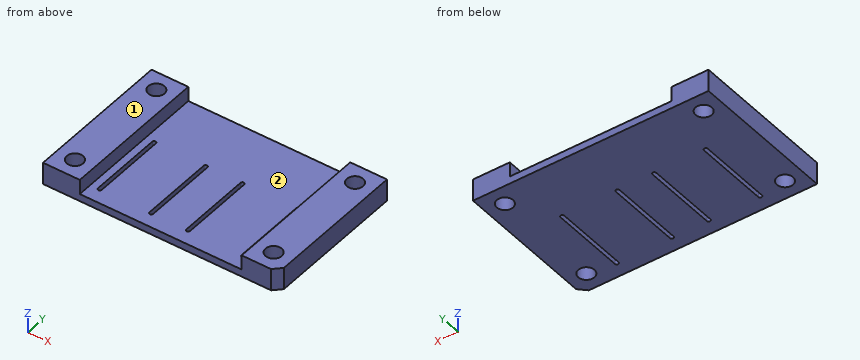
from build123d import *

# Parameters (mm, degrees)
SKETCH1_W           = 320
SKETCH1_H           = 200
SKETCH1_R           = 11
BOSS_EXTRUDE1_DEPTH = 30
CUT_EXTRUDE1_DEPTH  = 379.549864615
SKETCH4_W           = 220
SKETCH4_H           = 200
CUT_EXTRUDE2_DEPTH  = 20
CHAMFER1_SIZE       = 10


with BuildPart() as part:
    # Sketch1 → Boss-Extrude1 (new body)
    with BuildSketch(Plane.XY):
        with Locations((160, 100)):
            Rectangle(SKETCH1_W, SKETCH1_H)
        with Locations((25, 175)):
            Circle(SKETCH1_R, mode=Mode.SUBTRACT)
        with Locations((295, 175)):
            Circle(SKETCH1_R, mode=Mode.SUBTRACT)
        with Locations((25, 25)):
            Circle(SKETCH1_R, mode=Mode.SUBTRACT)
        with Locations((295, 25)):
            Circle(SKETCH1_R, mode=Mode.SUBTRACT)
    extrude(amount=BOSS_EXTRUDE1_DEPTH)

    # Sketch2 → Cut-Extrude1 (cut, through all)
    with BuildSketch(Plane.XY.offset(30)):
        with BuildLine():
            Line((260, 120), (260, 20))
            ThreePointArc((260, 20), (257.5, 17.5), (255, 20))
            Line((255, 20), (255, 120))
            ThreePointArc((255, 120), (257.5, 122.5), (260, 120))
        make_face()
        with BuildLine():
            Line((185, 120), (185, 20))
            ThreePointArc((185, 20), (182.5, 17.5), (180, 20))
            Line((180, 20), (180, 120))
            ThreePointArc((180, 120), (182.5, 122.5), (185, 120))
        make_face()
        with BuildLine():
            Line((65, 120), (65, 20))
            ThreePointArc((65, 20), (62.5, 17.5), (60, 20))
            Line((60, 20), (60, 120))
            ThreePointArc((60, 120), (62.5, 122.5), (65, 120))
        make_face()
        with BuildLine():
            Line((135, 120), (135, 20))
            ThreePointArc((135, 20), (132.5, 17.5), (130, 20))
            Line((130, 20), (130, 120))
            ThreePointArc((130, 120), (132.5, 122.5), (135, 120))
        make_face()
    extrude(amount=-CUT_EXTRUDE1_DEPTH, mode=Mode.SUBTRACT)

    # Sketch4 → Cut-Extrude2 (cut)
    with BuildSketch(Plane.XY.offset(30)):
        with Locations((160, 100)):
            Rectangle(SKETCH4_W, SKETCH4_H)
    extrude(amount=-CUT_EXTRUDE2_DEPTH, mode=Mode.SUBTRACT)

    # Chamfer1
    chamfer1_edges = [part.edges().sort_by_distance(p)[0] for p in [
        (320, 0, 15),
    ]]
    chamfer(chamfer1_edges, length=CHAMFER1_SIZE)


solid = part.part
The listing builds one solid part. Answer for the finished solid, in the listing's coordinates (mm). Face numbers are marked on the shaded views. A direction names the side the tool comes from. Give positions to 0.01 mm unless a question says otherwise; leave off trailing zeros. Write each loop counter-clockwise with the first axis right and the second up, starting at its lowest first coordinate (ties: lowest second). Pieces come first, ordered by that corner, then holes. Notation, with made-up numbers: (89.5, 55) - (124.5, 55) arc R15 ccw to (124.5, 59) - close; hole circle Ø2 at (5.5, -11.75). An arc over 180 degrees is marked (long way). Use a Markdown table: item, result.
1. Section B-B on z = 21 is taken. Write down the section's boundary in (x, y), plus the area to 3 significant figures.
Values follow:
| item | result |
|---|---|
| outline | (0, 0) - (50, 0) - (50, 200) - (0, 200) - close; (270, 0) - (310, 0) - (320, 10) - (320, 200) - (270, 200) - close; hole circle Ø22 at (25, 25); hole circle Ø22 at (25, 175); hole circle Ø22 at (295, 25); hole circle Ø22 at (295, 175) |
| area | 18,400 mm² |
2. Find the intervals of material crossed by probe 1 along Y at (x, z) = (25, 14.25); probe 2 along X at (y, z) = (142.5, 27.5); probe 3 along X at (y, z) = (25.5, 16), in increasing order. Write a range as from..to.
Values follow:
| item | result |
|---|---|
| probe 1 | y = 0..14, 36..164, 186..200 |
| probe 2 | x = 0..50, 270..320 |
| probe 3 | x = 0..14.01, 35.99..50, 270..284.01, 305.99..320 |
3. Each of these flat-tipped pins is pushed along its axis until it touches: P1, Ø12, axis at x = 131, y = 41, coming from the +Z side; P2, Ø16, axis at y = 137, z = 15, coming from the -X side; P3, Ø12, axis at x = 227, z = 19.5, coming from the -Y side. Where does it stop, or does it pass through?
Values follow:
| item | result |
|---|---|
| P1 | stops at z = 10 |
| P2 | stops at x = 0 |
| P3 | passes through |
4. Section C-C on y = 175 is taken. Write down the section's boundary in (x, z).
Values follow:
| item | result |
|---|---|
| outline | (0, 0) - (14, 0) - (14, 30) - (0, 30) - close; (36, 0) - (284, 0) - (284, 30) - (270, 30) - (270, 10) - (50, 10) - (50, 30) - (36, 30) - close; (306, 0) - (320, 0) - (320, 30) - (306, 30) - close |
5. A tool of negligible diameter and unlimited length cuts with its end or side. For the marked faces 1 and 2, from which of +Z, -Z, +X, -X, +Y, -Y can it reach the whole face along a straight path? Write none if from no direction.
Values follow:
| item | result |
|---|---|
| face 1 | +Z, +X, -X, +Y, -Y |
| face 2 | +Z, +Y, -Y |
6. Section A-A on y = 25 is taken. Count the separate pieces of the cut face and the enclosed holes in it, plus the area to 3 significant figures.
Values follow:
| item | result |
|---|---|
| separate pieces | 7 |
| enclosed holes | 0 |
| area | 3,680 mm² |
7. Section D-D on x = 25 is taken. Write down the section's boundary in (y, z), plus the area to 3 significant figures.
Values follow:
| item | result |
|---|---|
| outline | (0, 0) - (14, 0) - (14, 30) - (0, 30) - close; (36, 0) - (164, 0) - (164, 30) - (36, 30) - close; (186, 0) - (200, 0) - (200, 30) - (186, 30) - close |
| area | 4,680 mm² |
